Input: part model. Units: mm. Frame: model coordinates. A direction names the side the tool comes from. Round coordinates to 2 decimals unless told otherwise and drop trailing zeros. Loops run counter-clockwise (first coordinate to the right, second up) from the corner with the lowest first, then second, coordinate; pieces in that order, holes last. Notation, with made-up numbers: M 54.5,-19.75 L 108.5,-19.75 A18 cw 108.5,3.25 Z; hole C 34,24 d4. An arc over 180 degrees is marked long. Put each result on its own line as item: value. Start each with the question number.
1) Section C-C on x = 13. Output: boundary loops of the cut face in (y, z), plus the area to 3 significant figures.
2) Draft query along Z for faces 4 (the face through (-27, 4, 5)), 5 (the face through (24.54, -5.81, 5.38)), 6 (the face through (0, 0, 0)). Return one class per face: +Z half, -Z half, draft (parallel to the pull), parting line (faces both ways), or undercut.
3) Pin query (flat end, axial travel): pin 1 (2 mm diameter, centred on y = 7, z = 5, fed in from -X); pin 2 (5 mm diameter, centred on y = -1, z = 3.5, fed in from -X); pin 3 (1.5 mm diameter, centred on y = 0, z = 2.5, fed in from +X); pin 4 (3 mm diameter, centred on x = 6.5, z = 3.5, fed in from -Y). Return the tip coordinate at first contact, or that it passes through.
4) Line query: probe 1 along Y at (x, z) = (21.75, 5); probe 2 along Y at (x, z) = (-28.5, 5); probe 3 along Z at (x, y) = (23, 7). Output: solid intervals per line, ascending.
5) Section A-A on y = -4.75. Output: boundary loops of the cut face in (x, z), plus the area to 3 significant figures.
6) Section D-D on z = 5. State how many separate pieces and enclosed holes the cut face has, plus the area to 3 significant figures.
7) Reachability of faces 1 (the face through (17.82, -5.62, 4.93)), 2 (the face through (23, 0, 5)), 3 (the face through (20.01, 8.38, 3.82)) from +Z, -Z, +X, -X, +Y, -Y: full face, straight path, thin tool, end or side. Return the list, or none.
8) Section B-B on y = 7. Output: boundary loops of the cut face in (x, z), plus the area to 3 significant figures.
from build123d import *

# Parameters (mm, degrees)
F1_DEPTH = 10
F2_R     = 1.25
F3_DEPTH = 62.001


with BuildPart() as f1:
    # F0 (on Top) → F1 (new body)
    with BuildSketch(Plane.XY):
        Polygon((31, 4), (31, 10), (20.835134, 10), (17.777494, 4), (0, 4), (-17.777494, 4), (-20.835134, 10), (-31, 10), (-31, 4), (-23, 4), (-23, -4), (-31, -4), (-31, -10), (-20.350992, -10), (-16.88689, -4), (0, -4), (16.88689, -4), (20.350992, -10), (31, -10), (31, -4), (23, -4), (23, 4), align=None)
    extrude(amount=F1_DEPTH)

    # F2 (on face) → F3 (cut, through all)
    with BuildSketch(Plane.YZ.offset(31)):
        with Locations((-7, 5)):
            Circle(F2_R)
        with Locations((7, 5)):
            Circle(F2_R)
    extrude(amount=-F3_DEPTH, mode=Mode.SUBTRACT)


solid = f1.part
Geometry results:
1. outline: M -4,0 L 4,0 L 4,10 L -4,10 Z
1. area: 80.0 mm²
2. face 4: draft
2. face 5: undercut
2. face 6: -Z half
3. pin 1: passes through
3. pin 2: stops at x = -23
3. pin 3: stops at x = 23
3. pin 4: stops at y = -4
4. probe 1: y = -10 to -8.25, -5.75 to 5.75, 8.25 to 10
4. probe 2: y = -10 to -8.25, -5.75 to -4, 4 to 5.75, 8.25 to 10
4. probe 3: z = 0 to 3.75, 6.25 to 10
5. outline: M -31,0 L -17.32,0 L -17.32,10 L -31,10 Z; M 17.32,0 L 31,0 L 31,10 L 17.32,10 Z
5. area: 274 mm²
6. separate pieces: 5
6. enclosed holes: 0
6. area: 537 mm²
7. face 1: +Z, -Z, -Y
7. face 2: +Z, -Z, +X
7. face 3: +Z, -Z, +Y
8. outline: M -31,0 L -19.31,0 L -19.31,3.75 L -31,3.75 Z; M -31,6.25 L -19.31,6.25 L -19.31,10 L -31,10 Z; M 19.31,0 L 31,0 L 31,3.75 L 19.31,3.75 Z; M 19.31,6.25 L 31,6.25 L 31,10 L 19.31,10 Z
8. area: 175 mm²
